Geometry: final body of the model. Coordinates: model frame, mm. A direction names the side the tool comes from. Round coordinates to 2 decimals unless told otherwise and drop trailing zeros. Order: outer loops, then holes, each group sorted by start corner. A loop starts at its lowest first (then second) coordinate and runs counter-clockwise, first axis right, second up. Notation, with made-up numbers: (74, 82.25) - (113, 82.25) arc R15 cw to (113, 88.25) - close; hole circle Ø3 at (-1.5, 23). An arc over 180 degrees is marked (long way). Put each result on its own line as item: value. Start each with the question number.
(1) Pin query (flat end, axial travel): P1, Ø6, axis at x = -13, z = 0, coming from the -Y side; P2, Ø1, axis at x = -11.5, y = 0.5, coming from the +Z side; P3, Ø2, axis at x = -1, z = -1.5, coming from the -Y side; P4, Ø4.5, axis at x = 2, z = -2, coming from the +Y side. Return the tip coordinate at first contact, or that it passes through.
(2) Section B-B (y = 2.25). Output: boundary loops of the cut face in (x, z), and give its area (3 significant figures).
(3) Section D-D (z = -3). Output: boundary loops of the cut face in (x, y), and give its area (3 significant figures).
(4) Material intervals for L1, parallel to Y at x = 4, z = 0; L2, parallel to Y at x = -14, z = -4, sorted ascending. Write a range as [from, to].
(5) Access query for faces 4 (the face through (0.45, 2.01, -1.43)), 5 (the face through (-3.417, -0.268, 0.759)), 6 (the face through (16, 0, 0)), 7 (the face through (1.352, 5.219, 4.292)). Directions: +Z, -Z, +X, -X, +Y, -Y. A direction counts if a zero-diameter tool reaches every point of the face in a straight line with its end or side. Return the directions, or none.
(6) Pull-direction query (Z, two-part tool) for faces 1 (the face through (24.737, 1.521, 0.195)), 2 (the face through (-16, 0, 0)), 3 (the face through (-27, 1, 0)); classes: released by +Z, released by -Z, zero draft, split by the parting line, or undercut.
(7) Section C-C (y = 5). Output: boundary loops of the cut face in (x, z).
from build123d import *
from build123d.topology import SkipClean

# Parameters (mm, degrees)
SALIENTE_EXTRUIR1_DEPTH             = 3
CROQUIS2_R                          = 6.5
CROQUIS2_R_2                        = 4.5
SALIENTE_EXTRUIR2_DEPTH             = 4.5
SALIENTE_EXTRUIR3_START             = 1.5
SALIENTE_EXTRUIR3_DEPTH             = 1.5
SALIENTE_EXTRUIR4_REACH             = 30.766
SALIENTE_EXTRUIR4_DIRECTION_2_REACH = 30.766
SALIENTE_EXTRUIR5_REACH             = 30.766
SALIENTE_EXTRUIR5_DIRECTION_2_REACH = 30.766
CROQUIS7_R                          = 3.5
CORTAR_EXTRUIR1_DEPTH               = 2.5
CORTAR_EXTRUIR2_DEPTH               = 29.521921394
CORTAR_EXTRUIR2_DEPTH_BACK          = 29.521921394
CROQUIS8_R                          = 1.5


with BuildPart() as part:
    # Croquis1 → Saliente-Extruir1 (new body)
    with BuildSketch(Plane(origin=(0, 0, 0), x_dir=(1, 0, 0), z_dir=(0, 1, 0))):
        with BuildLine():
            Line((0.768817204, 6.45437217), (23.693548387, 3.723676252))
            ThreePointArc((23.693548387, 3.723676252), (27, 0), (23.693548387, -3.723676252))
            Line((23.693548387, -3.723676252), (0.768817204, -6.45437217))
            ThreePointArc((0.768817204, -6.45437217), (0, -6.5), (-0.768817204, -6.45437217))
            Line((-0.768817204, -6.45437217), (-23.693548387, -3.723676252))
            ThreePointArc((-23.693548387, -3.723676252), (-27, 0), (-23.693548387, 3.723676252))
            Line((-23.693548387, 3.723676252), (-0.768817204, 6.45437217))
            ThreePointArc((-0.768817204, 6.45437217), (0, 6.5), (0.768817204, 6.45437217))
        make_face()
    extrude(amount=SALIENTE_EXTRUIR1_DEPTH)

    # Croquis2 → Saliente-Extruir2 (add)
    with BuildSketch(Plane(origin=(0, 3, 0), x_dir=(1, 0, 0), z_dir=(0, 1, 0))):
        with Locations(Location((0, 0, 0), (0, 0, 83.207177944))):
            Circle(CROQUIS2_R)
        with Locations(Location((0, 0, 0), (0, 0, 270))):
            Circle(CROQUIS2_R_2, mode=Mode.SUBTRACT)
    extrude(amount=SALIENTE_EXTRUIR2_DEPTH)

    # Croquis3 → Saliente-Extruir3 (add)
    with SkipClean():  # the faces are left unmerged after this step: merging them gives an invalid solid
        with BuildSketch(Plane.XZ.offset(SALIENTE_EXTRUIR3_START)):
            with BuildLine():
                Line((4, -6.069487497), (0.768817204, -6.45437217))
                ThreePointArc((0.768817204, -6.45437217), (0, -6.5), (-0.768817204, -6.45437217))
                Line((-0.768817204, -6.45437217), (-4, -6.069487497))
                Line((-4, -6.069487497), (-4, 6.069487497))
                Line((-4, 6.069487497), (-0.768817204, 6.45437217))
                ThreePointArc((-0.768817204, 6.45437217), (0, 6.5), (0.768817204, 6.45437217))
                Line((0.768817204, 6.45437217), (4, 6.069487497))
                Line((4, 6.069487497), (4, -6.069487497))
            make_face()
        extrude(amount=-SALIENTE_EXTRUIR3_DEPTH)

    # Saliente-Extruir4: up to this plane
    with SkipClean():  # the faces are left unmerged after this step: merging them gives an invalid solid
        saliente_extruir4_end = Plane(origin=(-0.768817204, 3, 6.45437217), z_dir=(0.11827956989247339, 0, -0.992980333816361))
        # Croquis4 → Saliente-Extruir4 (add, up to the surface)
        with BuildSketch(Plane.XY, mode=Mode.PRIVATE) as saliente_extruir4_sk1:
            Polygon((-4, -1.5), (-4, 0), (-9, 0), align=None)
        saliente_extruir4_tool1 = split(extrude(saliente_extruir4_sk1.sketch, amount=SALIENTE_EXTRUIR4_REACH, mode=Mode.PRIVATE), bisect_by=saliente_extruir4_end, keep=Keep.BOTH, mode=Mode.PRIVATE)
        add(saliente_extruir4_tool1.solids().sort_by_distance((-5.666667, -0.5, 0))[0])

    # Saliente-Extruir4 direction 2: up to this plane
    with SkipClean():  # the faces are left unmerged after this step: merging them gives an invalid solid
        saliente_extruir4_direction_2_end = Plane(origin=(-0.768817204, 3, -6.45437217), z_dir=(0.11827956989247339, 0, 0.992980333816361))
        # Croquis4 → Saliente-Extruir4 direction 2 (add, up to the surface)
        with BuildSketch(Plane.XY, mode=Mode.PRIVATE) as saliente_extruir4_direction_2_sk1:
            Polygon((-4, -1.5), (-4, 0), (-9, 0), align=None)
        saliente_extruir4_direction_2_tool1 = split(extrude(saliente_extruir4_direction_2_sk1.sketch, amount=-SALIENTE_EXTRUIR4_DIRECTION_2_REACH, mode=Mode.PRIVATE), bisect_by=saliente_extruir4_direction_2_end, keep=Keep.BOTH, mode=Mode.PRIVATE)
        add(saliente_extruir4_direction_2_tool1.solids().sort_by_distance((-5.666667, -0.5, 0))[0])

    # Saliente-Extruir5: up to this plane
    with SkipClean():  # the faces are left unmerged after this step: merging them gives an invalid solid
        saliente_extruir5_end = Plane(origin=(0.768817204, 3, 6.45437217), z_dir=(-0.11827956989247339, 0, -0.992980333816361))
        # Croquis5 → Saliente-Extruir5 (add, up to the surface)
        with BuildSketch(Plane.XY, mode=Mode.PRIVATE) as saliente_extruir5_sk1:
            Polygon((4, 0), (9, 0), (4, -1.5), align=None)
        saliente_extruir5_tool1 = split(extrude(saliente_extruir5_sk1.sketch, amount=SALIENTE_EXTRUIR5_REACH, mode=Mode.PRIVATE), bisect_by=saliente_extruir5_end, keep=Keep.BOTH, mode=Mode.PRIVATE)
        add(saliente_extruir5_tool1.solids().sort_by_distance((5.666667, -0.5, 0))[0])

    # Saliente-Extruir5 direction 2: up to this plane
    with SkipClean():  # the faces are left unmerged after this step: merging them gives an invalid solid
        saliente_extruir5_direction_2_end = Plane(origin=(0.768817204, 3, -6.45437217), z_dir=(-0.11827956989247339, 0, 0.992980333816361))
        # Croquis5 → Saliente-Extruir5 direction 2 (add, up to the surface)
        with BuildSketch(Plane.XY, mode=Mode.PRIVATE) as saliente_extruir5_direction_2_sk1:
            Polygon((4, 0), (9, 0), (4, -1.5), align=None)
        saliente_extruir5_direction_2_tool1 = split(extrude(saliente_extruir5_direction_2_sk1.sketch, amount=-SALIENTE_EXTRUIR5_DIRECTION_2_REACH, mode=Mode.PRIVATE), bisect_by=saliente_extruir5_direction_2_end, keep=Keep.BOTH, mode=Mode.PRIVATE)
        add(saliente_extruir5_direction_2_tool1.solids().sort_by_distance((5.666667, -0.5, 0))[0])

    # Croquis7 → Cortar-Extruir1 (cut)
    with SkipClean():  # the faces are left unmerged after this step: merging them gives an invalid solid
        with BuildSketch(Plane.XZ.offset(1.5)):
            with Locations(Location((0, 0, 0), (0, 0, 270))):
                Circle(CROQUIS7_R)
        extrude(amount=-CORTAR_EXTRUIR1_DEPTH, mode=Mode.SUBTRACT)

    # Croquis8 → Cortar-Extruir2 (cut, two sides: drawn at the far end of the back side and taken through both)
    with SkipClean():  # the faces are left unmerged after this step: merging them gives an invalid solid
        with BuildSketch(Plane.XZ.offset(-1).offset(-CORTAR_EXTRUIR2_DEPTH_BACK)):
            with Locations(Location((0, 0, 0), (0, 0, 270))):
                Circle(CROQUIS8_R)
            with Locations(Location((12.25, 0, 0), (0, 0, 270))):
                Circle(CROQUIS8_R)
            with Locations(Location((17.75, 0, 0), (0, 0, 270))):
                Circle(CROQUIS8_R)
            with Locations(Location((23.25, 0, 0), (0, 0, 270))):
                Circle(CROQUIS8_R)
            with Locations(Location((-23.25, 0, 0), (0, 0, 270))):
                Circle(CROQUIS8_R)
            with Locations(Location((-17.75, 0, 0), (0, 0, 270))):
                Circle(CROQUIS8_R)
            with Locations(Location((-12.25, 0, 0), (0, 0, 270))):
                Circle(CROQUIS8_R)
        extrude(amount=CORTAR_EXTRUIR2_DEPTH + CORTAR_EXTRUIR2_DEPTH_BACK, mode=Mode.SUBTRACT)


solid = part.part
Checks:
1. P1: stops at y = 0
1. P2: stops at z = 5.24
1. P3: stops at y = 1
1. P4: stops at y = 7.5
2. outline: (-23.69, -3.72) - (-0.77, -6.45) arc R6.5 ccw to (0.77, -6.45) - (23.69, -3.72) arc R3.75 ccw to (23.69, 3.72) - (0.77, 6.45) arc R6.5 ccw to (-0.77, 6.45) - (-23.69, 3.72) arc R3.75 ccw to start; hole circle Ø3 at (-23.25, 0); hole circle Ø3 at (-17.75, 0); hole circle Ø3 at (-12.25, 0); hole circle Ø3 at (0, 0); hole circle Ø3 at (12.25, 0); hole circle Ø3 at (17.75, 0); hole circle Ø3 at (23.25, 0)
2. area: 475 mm²
3. outline: (-25.5, 0) - (-9, 0) - (-4, -1.5) - (-1.8, -1.5) - (-1.8, 1) - (1.8, 1) - (1.8, -1.5) - (4, -1.5) - (9, 0) - (25.5, 0) - (25.5, 3) - (5.77, 3) - (5.77, 7.5) - (3.35, 7.5) - (3.35, 3) - (-3.35, 3) - (-3.35, 7.5) - (-5.77, 7.5) - (-5.77, 3) - (-25.5, 3) - close
3. area: 185 mm²
4. L1: y = [-1.5, 3]
4. L2: y = [0, 3]
5. face 4: +Y, -Y
5. face 5: -Y
5. face 6: +Z, -Z, +X, -Y
5. face 7: +Y
6. face 1: undercut
6. face 2: zero draft
6. face 3: split by the parting line
7. outline: circle Ø13 at (0, 0); hole circle Ø9 at (0, 0)
